Study the drawing (mm; zero at the part's minimum x, y, z) and answer. A direction names the side the tool comes from. Give positions to 0.01 mm unless a question says otherwise; leave off trailing zeros. Loops run counter-clockwise (first coordinate to the right, second up) from the corner with the lowest first, then second, coordinate; pieces in that order, holes last. Notation, with made-up numbers: (27.25, 37.25) - (32.25, 37.25) arc R32 cw to (32.25, 69.25) - close; hole circle Ø1 at (1, 8). An arc over 180 degrees is marked (long way). Write item = value, one per line. Start each with the question number.
1) The part is cut by section B-B on y = 39. Write down the section's boundary in (x, z).
2) The part is cut by section C-C on z = 6. Write down the section's boundary in (x, y).
3) The part is cut by section A-A on x = 7. Write down the section's boundary in (y, z), plus the area to 3 significant figures.
4) Which of the six approach directions +Z, -Z, +X, -X, +Y, -Y give full straight-line access (tool end or side, diameter ignored) to the marked faces 1, 2 and 3?
5) Flat-ended cylindrical pins translate along their axes: P1, Ø12, axis at x = 31.5, y = 18, coming from the +Z side; P2, Ø5, axis at x = 20, y = 16, coming from the -Z side; P3, Ø10, axis at y = 24, z = 45.5, coming from the +X side; P4, Ø5, axis at x = 99, z = 14.5, coming from the -Y side. Find the tip coordinate at first contact, or state that the pin passes through.
6) The part is cut by section D-D on y = 14.5. Write down the section's boundary in (x, z).
7) Consider probe 1 along X at (y, z) = (36, 19); probe 2 along Z at (x, y) = (9, 30); probe 3 along X at (y, z) = (22, 11.5). Determine where each line is inside the solid, lowest interval first.
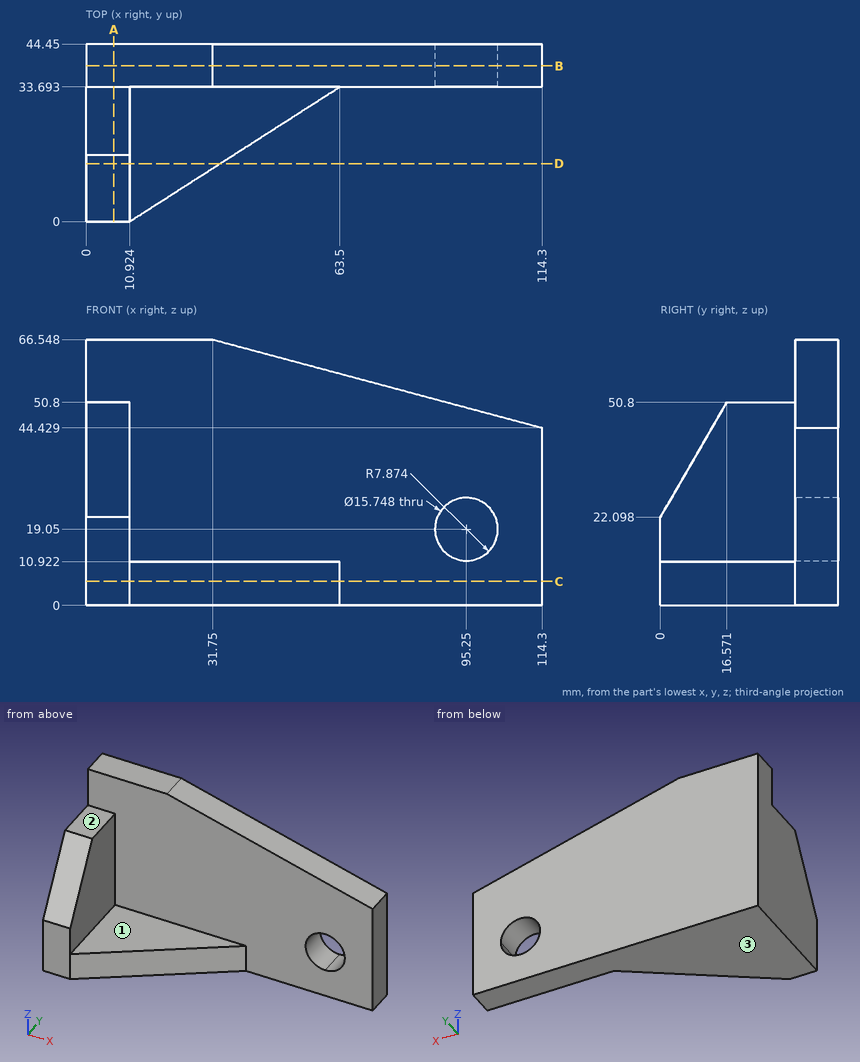
Answer below:
q1.outline = (0, 0) - (114.3, 0) - (114.3, 44.43) - (31.75, 66.55) - (0, 66.55) - close; hole circle Ø15.75 at (95.25, 19.05)
q2.outline = (0, 0) - (10.92, 0) - (63.5, 33.69) - (114.3, 33.69) - (114.3, 44.45) - (0, 44.45) - close
q3.outline = (0, 0) - (44.45, 0) - (44.45, 66.55) - (33.69, 66.55) - (33.69, 50.8) - (16.57, 50.8) - (0, 22.1) - close
q3.area = 2,190 mm2
q4.face_1 = +Z, +X, -Y
q4.face_2 = +Z, +X, -X, -Y
q4.face_3 = -Z, +X, -X, +Y, -Y
q5.P1 = 10.92
q5.P2 = 0
q5.P3 = 10.92
q5.P4 = 33.69
q6.outline = (0, 0) - (33.55, 0) - (33.55, 10.92) - (10.92, 10.92) - (10.92, 47.21) - (0, 47.21) - close
q7.probe_1 = 0 to 87.38, 103.12 to 114.3
q7.probe_2 = 0 to 50.8
q7.probe_3 = 0 to 10.92
